Here's how the part is built. I have some questions about the finished solid (model axes, mm). A direction names the side the tool comes from. Coordinates: 2 decimals unless noted, no trailing zeros. Answer as CSV lines item,"result". Start each with the question number.
Q1. I need wall thicknesses on line 1 (Y direction, x = 4.35, z = -85); line 2 (Y direction, x = -3.25, z = 103); line 3 (X direction, y = 19.5, z = 108). Which ranges of each line are inside material? Lowest first, please.
Q2. Thinking about a two-plate mould opening in Y: for faces 1 (the face through (2, -20, 2)), 2 (the face through (-4.493, -0.402, 17.101)), 3 (the face through (0.09, -19.49, 90.9)), which applies, released by +Y, released by -Y, zero draft, split by the parting line, or undercut?
Q3. For faces 4 (the face through (-4, -9, 2)), 5 (the face through (4.49, -0.21, -17.39)), 6 (the face through (2.033, -19.507, 0.267)), which set-ups out of +Z, -Z, +X, -X, +Y, -Y let a thin tool reach every point of the face, with its end or its side?
Q4. Suppose I cut it at A-A (z = 15). Count the separate pieces of the cut face and the enclosed holes in it, then the cut area to 3 significant figures.
from build123d import *

# Parameters (mm, degrees)
SKETCH_1_W          = 10
SKETCH_1_H          = 40
SKETCH_1_W_2        = 8
SKETCH_1_H_2        = 38
EXTRUDE_1_DEPTH     = 113
SKETCH_3_R          = 2.1
CUT_EXTRUDE_1_DEPTH = 15
SKETCH_5_R          = 2.1
CUT_EXTRUDE_3_DEPTH = 25
CUT_EXTRUDE_4_DEPTH = 25
FILLET_3_R          = 1.5
FILLET_4_R          = 1.5
SKETCH_10_R         = 11
CUT_EXTRUDE_6_DEPTH = 25
CUT_EXTRUDE_7_REACH = 121.975
SKETCH_11_R         = 2.05
SKETCH_12_R         = 2.1
CUT_EXTRUDE_8_DEPTH = 120.974997395
SKETCH_15_R         = 2.1
SKETCH_15_R_2       = 1.7
CUT_EXTRUDE_9_DEPTH = 116.331045257


with BuildPart() as part:
    # 草图1 → 凸台-拉伸1 (new, symmetric)
    with BuildSketch(Plane.XY):
        Rectangle(SKETCH_1_W, SKETCH_1_H)
        Rectangle(SKETCH_1_W_2, SKETCH_1_H_2, mode=Mode.SUBTRACT)
    extrude(amount=EXTRUDE_1_DEPTH, both=True)

    # 草图3 → 切除-拉伸1 (cut, symmetric)
    with BuildSketch(Plane(origin=(0, 0, 0), x_dir=(0, 0, -1), z_dir=(1, 0, 0))):
        with Locations(Location((30, 15, 0), (0, 0, 270))):
            Circle(SKETCH_3_R)
        with Locations(Location((-30, 15, 0), (0, 0, 270))):
            Circle(SKETCH_3_R)
        with Locations(Location((0, -15, 0), (0, 0, 270))):
            Circle(SKETCH_3_R)
    extrude(amount=CUT_EXTRUDE_1_DEPTH, both=True, mode=Mode.SUBTRACT)

    # 草图5 → 切除-拉伸3 (cut, symmetric)
    with BuildSketch(Plane(origin=(0, 0, 0), x_dir=(1, 0, 0), z_dir=(0, 1, 0))):
        with Locations(Location((0, 15, 0), (0, 0, 90))):
            Circle(SKETCH_5_R)
        with Locations(Location((0, 45, 0), (0, 0, 90))):
            Circle(SKETCH_5_R)
        with Locations(Location((0, -45, 0), (0, 0, 90))):
            Circle(SKETCH_5_R)
        with Locations(Location((0, -15, 0), (0, 0, 90))):
            Circle(SKETCH_5_R)
    extrude(amount=CUT_EXTRUDE_3_DEPTH, both=True, mode=Mode.SUBTRACT)

    # 草图7 → 切除-拉伸4 (cut, symmetric)
    with BuildSketch(Plane(origin=(0, 0, 0), x_dir=(0, 0, -1), z_dir=(1, 0, 0))):
        Polygon((-1.5, -7.197224362), (-1.5, 10), (-27.295836543, 10), align=None)
        Polygon((27.295836543, 10), (1.5, 10), (1.5, -7.197224362), align=None)
        Polygon((30, 8.197224362), (2.704163457, -10), (30, -10), align=None)
        Polygon((-30, -10), (-2.704163457, -10), (-30, 8.197224362), align=None)
    extrude(amount=CUT_EXTRUDE_4_DEPTH, both=True, mode=Mode.SUBTRACT)

    # 圆角3
    fillet_3_edges = [part.edges().sort_by_distance(p)[0] for p in [
        (4.5, 8.197224362, 30),
        (4.5, -10, 2.704163457),
        (4.5, -10, 30),
        (4.5, 10, -27.295836543),
        (4.5, -7.197224362, -1.5),
        (4.5, 10, -1.5),
        (4.5, 8.197224362, -30),
        (4.5, -10, -30),
        (4.5, -10, -2.704163457),
        (4.5, 10, 1.5),
        (4.5, -7.197224362, 1.5),
        (4.5, 10, 27.295836543),
    ]]
    fillet(fillet_3_edges, radius=FILLET_3_R)

    # 圆角4
    fillet_4_edges = [part.edges().sort_by_distance(p)[0] for p in [
        (-4.5, 8.197224362, 30),
        (-4.5, -10, 2.704163457),
        (-4.5, -10, 30),
        (-4.5, 10, -27.295836543),
        (-4.5, -7.197224362, -1.5),
        (-4.5, 10, -1.5),
        (-4.5, 8.197224362, -30),
        (-4.5, -10, -30),
        (-4.5, -10, -2.704163457),
        (-4.5, 10, 1.5),
        (-4.5, -7.197224362, 1.5),
        (-4.5, 10, 27.295836543),
    ]]
    fillet(fillet_4_edges, radius=FILLET_4_R)

    # 草图10 → 切除-拉伸6 (cut, symmetric)
    with BuildSketch(Plane(origin=(0, 0, 0), x_dir=(0, 0, -1), z_dir=(1, 0, 0))):
        with Locations(Location((-85, 0, 0), (0, 0, 270))):
            Circle(SKETCH_10_R)
        with Locations(Location((-55, 0, 0), (0, 0, 270))):
            Circle(SKETCH_10_R)
        with Locations(Location((55, 0, 0), (0, 0, 270))):
            Circle(SKETCH_10_R)
        with Locations(Location((85, 0, 0), (0, 0, 270))):
            Circle(SKETCH_10_R)
    extrude(amount=CUT_EXTRUDE_6_DEPTH, both=True, mode=Mode.SUBTRACT)

    # 草图11 → 切除-拉伸7 (cut, up to next)
    with BuildSketch(Plane.XZ.offset(20), mode=Mode.PRIVATE) as cut_extrude_7_sk1:
        with Locations(Location((0, 0, 0), (0, 0, 270))):
            Circle(SKETCH_11_R)
    cut_extrude_7_tool1 = extrude(cut_extrude_7_sk1.sketch, amount=-CUT_EXTRUDE_7_REACH, mode=Mode.PRIVATE) & part.part
    add(cut_extrude_7_tool1.solids().sort_by_distance((0, -20, 0))[0], mode=Mode.SUBTRACT)

    # 草图12 → 切除-拉伸8 (cut, through all)
    with BuildSketch(Plane(origin=(0, 20, 0), x_dir=(1, 0, 0), z_dir=(0, 1, 0))):
        with Locations(Location((0, 108, 0), (0, 0, 270))):
            Circle(SKETCH_12_R)
        with Locations(Location((0, 93, 0), (0, 0, 270))):
            Circle(SKETCH_12_R)
        with Locations(Location((0, -108, 0), (0, 0, 270))):
            Circle(SKETCH_12_R)
        with Locations(Location((0, -93, 0), (0, 0, 270))):
            Circle(SKETCH_12_R)
    extrude(amount=-CUT_EXTRUDE_8_DEPTH, mode=Mode.SUBTRACT)

    # 草图15 → 切除-拉伸9 (cut, through all)
    with BuildSketch(Plane(origin=(6.5, 0, 0), x_dir=(0, 0, -1), z_dir=(1, 0, 0))):
        with Locations(Location((0, -15, 0), (0, 0, 270))):
            Circle(SKETCH_15_R)
        with Locations(Location((30, 15, 0), (0, 0, 270))):
            Circle(SKETCH_15_R)
        with Locations(Location((-30, 15, 0), (0, 0, 270))):
            Circle(SKETCH_15_R)
        with Locations(Location((-37, 0, 0), (0, 0, 270))):
            Circle(SKETCH_15_R_2)
        with Locations(Location((37, 0, 0), (0, 0, 270))):
            Circle(SKETCH_15_R_2)
        with Locations(Location((70, 0, 0), (0, 0, 270))):
            Circle(SKETCH_15_R_2)
        with Locations(Location((-109.5, 0, 0), (0, 0, 270))):
            Circle(SKETCH_15_R_2)
        with Locations(Location((-85, -15, 0), (0, 0, 270))):
            Circle(SKETCH_15_R_2)
        with Locations(Location((109.5, 0, 0), (0, 0, 270))):
            Circle(SKETCH_15_R_2)
        with Locations(Location((-55, 15, 0), (0, 0, 270))):
            Circle(SKETCH_15_R_2)
        with Locations(Location((-70, 0, 0), (0, 0, 270))):
            Circle(SKETCH_15_R_2)
        with Locations(Location((55, 15, 0), (0, 0, 270))):
            Circle(SKETCH_15_R_2)
        with Locations(Location((-55, -15, 0), (0, 0, 270))):
            Circle(SKETCH_15_R_2)
        with Locations(Location((85, 15, 0), (0, 0, 270))):
            Circle(SKETCH_15_R_2)
        with Locations(Location((-85, 15, 0), (0, 0, 270))):
            Circle(SKETCH_15_R_2)
        with Locations(Location((55, -15, 0), (0, 0, 270))):
            Circle(SKETCH_15_R_2)
        with Locations(Location((85, -15, 0), (0, 0, 270))):
            Circle(SKETCH_15_R_2)
    extrude(amount=-CUT_EXTRUDE_9_DEPTH, mode=Mode.SUBTRACT)


solid = part.part
Here are the results:
1,line 1,"y = -20 to -16.7, -13.3 to -11, 11 to 13.3, 16.7 to 20"
1,line 2,"y = -20 to -19, 19 to 20"
1,line 3,"x = -5 to -2.1, 2.1 to 5"
2,face 1,"released by -Y"
2,face 2,"undercut"
2,face 3,"zero draft"
3,face 4,"+Z, -Z"
3,face 5,"+X, -X"
3,face 6,"-Y"
4,separate pieces,"6"
4,enclosed holes,"0"
4,area,"54.8 mm²"
